```python
from build123d import *

# Parameters (mm, degrees)
CROQUIS1_W              = 160
CROQUIS1_H              = 400
SALIENTE_EXTRUIR1_DEPTH = 400
REDONDEO1_R             = 5
CROQUIS2_R              = 15
CROQUIS2_R_2            = 5
CROQUIS2_W              = 150
CROQUIS2_H              = 40
CROQUIS2_W_2            = 105.514825976
CROQUIS2_H_2            = 8
CORTAR_EXTRUIR1_DEPTH   = 2
CROQUIS3_R              = 12.203694642
CROQUIS3_R_2            = 4.521298069
SALIENTE_EXTRUIR2_DEPTH = 5
CROQUIS4_W              = 380
CROQUIS4_H              = 380
CORTAR_EXTRUIR2_DEPTH   = 2
CROQUIS5_W              = 380
CROQUIS5_H              = 380
CORTAR_EXTRUIR3_DEPTH   = 2


with BuildPart() as part:
    # Croquis1 → Saliente-Extruir1 (new body)
    with BuildSketch(Plane.XY):
        Rectangle(CROQUIS1_W, CROQUIS1_H)
    extrude(amount=-SALIENTE_EXTRUIR1_DEPTH)

    # Redondeo1
    redondeo1_edges = [part.edges().sort_by_distance(p)[0] for p in [
        (80, 0, -400),
        (0, 200, -400),
        (-80, 0, -400),
        (0, 200, 0),
        (80, 0, 0),
        (0, -200, 0),
        (-80, 0, 0),
        (0, -200, -400),
        (-80, 200, -200),
        (80, 200, -200),
        (80, -200, -200),
        (-80, -200, -200),
    ]]
    fillet(redondeo1_edges, radius=REDONDEO1_R)

    # Croquis2 → Cortar-Extruir1 (cut)
    with BuildSketch(Plane.XY):
        with Locations((-42.906419047, -77.137880051)):
            Circle(CROQUIS2_R)
        with Locations((-10.118013228, -77.137880051)):
            Circle(CROQUIS2_R_2)
        with Locations((0, 175)):
            Rectangle(CROQUIS2_W, CROQUIS2_H)
        with Locations((0, 125)):
            Rectangle(CROQUIS2_W, CROQUIS2_H)
        with Locations((0, 35)):
            Rectangle(CROQUIS2_W, CROQUIS2_H)
        with Locations((-0.46526055, -176)):
            Rectangle(CROQUIS2_W_2, CROQUIS2_H_2)
        with Locations((-0.46526055, -158)):
            Rectangle(CROQUIS2_W_2, CROQUIS2_H_2)
        with Locations((-0.46526055, -140)):
            Rectangle(CROQUIS2_W_2, CROQUIS2_H_2)
    extrude(amount=-CORTAR_EXTRUIR1_DEPTH, mode=Mode.SUBTRACT)

    # Croquis3 → Saliente-Extruir2 (add)
    with BuildSketch(Plane.XY.offset(-2)):
        with Locations((-42.906419047, -77.137880051)):
            Circle(CROQUIS3_R)
        with Locations((-10.118013228, -77.137880051)):
            Circle(CROQUIS3_R_2)
    extrude(amount=SALIENTE_EXTRUIR2_DEPTH)

    # Croquis4 → Cortar-Extruir2 (cut)
    with BuildSketch(Plane.ZY.offset(80)):
        with Locations((-200, 0)):
            Rectangle(CROQUIS4_W, CROQUIS4_H)
    extrude(amount=-CORTAR_EXTRUIR2_DEPTH, mode=Mode.SUBTRACT)

    # Croquis5 → Cortar-Extruir3 (cut)
    with BuildSketch(Plane(origin=(80, 0, 0), x_dir=(0, 0, -1), z_dir=(1, 0, 0))):
        with Locations((200, 0)):
            Rectangle(CROQUIS5_W, CROQUIS5_H)
    extrude(amount=-CORTAR_EXTRUIR3_DEPTH, mode=Mode.SUBTRACT)


solid = part.part
```
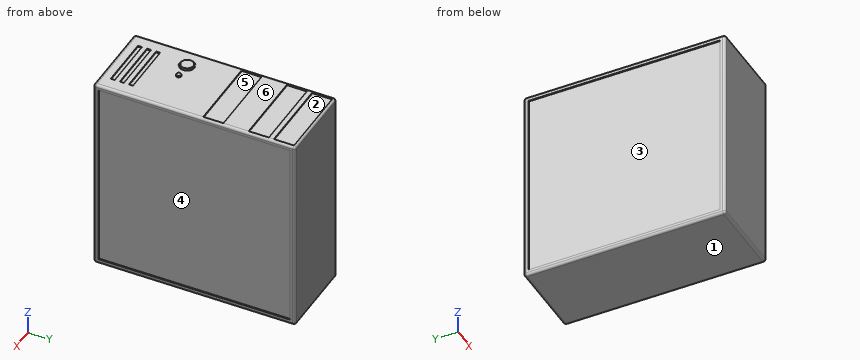
The model under review builds one solid part; all positions refer to its coordinate system, in mm. Face numbers are marked on the shaded views. A direction names the side the tool comes from. Give positions to 0.01 mm unless a question says otherwise; leave off trailing zeros. Write each loop counter-clockwise with the first axis right and the second up, starting at its lowest first coordinate (ties: lowest second). Pieces come first, ordered by that corner, then holes. Notation, with made-up numbers: (-25.5, 46.25) - (1.5, 46.25) arc R18 ccw to (1.5, 57.25) - close; hole circle Ø7 at (84, 38.25). An arc over 180 degrees is marked (long way). Answer in a Markdown table with one row per item. Add a question column.
1. We need section A-A on z = -314. Write out the cut boundary in (x, y).
2. Wall thickness on line 1 along X through (y, z) = (-155, -345); line 2 along Z through (x, y) = (23, -45); line 3 along Z through (x, y) = (9, 138.5): over which ranges is each line inside the solid? List them lowest first. Write a range as [from, to].
3. We need section B-B on y = 94.5. Write out the cut boundary in (x, z).
4. Tool access review of the marked faces 4, 5 and 6: name each direction out of +Z, -Z, +X, -X, +Y, -Y from which nothing blocks a thin tool from reaching the whole face with its end or side.
5. We need section C-C on y = 25.5. Write out the cut boundary in (x, z), then the cut area to 3 significant figures.
6. Insertion check: P1, Ø1, axis at y = -27.5, z = -190, coming from the -X side; P2, Ø1, axis at x = 79, y = 70, coming from the +Z side; P3, Ø2, axis at y = 176, z = -1.5, coming from the -X side. Each pin has a flat end and moves straight along its axis. Give the tip position at first contact, or say it passes through.
7. Draft analysis for pull direction X (two halves, no side actions). For the marked faces 1, 2 and 3, state which applies: +X half, -X half, draft (parallel to the pull), parting line (faces both ways), or undercut.
Ans:
| question | item | result |
|---|---|---|
| 1 | outline | (-80, -195) arc R5 ccw to (-75, -200) - (75, -200) arc R5 ccw to (80, -195) - (80, -190) - (78, -190) - (78, 190) - (80, 190) - (80, 195) arc R5 ccw to (75, 200) - (-75, 200) arc R5 ccw to (-80, 195) - (-80, 190) - (-78, 190) - (-78, -190) - (-80, -190) - close |
| 2 | line 1 | x = [-78, 78] |
| 2 | line 2 | z = [-400, 0] |
| 2 | line 3 | z = [-400, -2] |
| 3 | outline | (-80, -395) arc R5 ccw to (-75, -400) - (75, -400) arc R5 ccw to (80, -395) - (80, -390) - (78, -390) - (78, -10) - (80, -10) - (80, -5) arc R5 ccw to (75, 0) - (-75, 0) arc R5 ccw to (-80, -5) - (-80, -10) - (-78, -10) - (-78, -390) - (-80, -390) - close |
| 4 | face 4 | +X |
| 4 | face 5 | +Z |
| 4 | face 6 | +Z, +X, -X, +Y |
| 5 | outline | (-80, -395) arc R5 ccw to (-75, -400) - (75, -400) arc R5 ccw to (80, -395) - (80, -390) - (78, -390) - (78, -10) - (80, -10) - (80, -5) arc R5 ccw to (75, 0) - (75, -2) - (-75, -2) - (-75, 0) arc R5 ccw to (-80, -5) - (-80, -10) - (-78, -10) - (-78, -390) - (-80, -390) - close |
| 5 | area | 62,200 mm^2 |
| 6 | P1 | stops at x = -78 |
| 6 | P2 | stops at z = -1.43 |
| 6 | P3 | stops at x = -79.33 |
| 7 | face 1 | draft |
| 7 | face 2 | undercut |
| 7 | face 3 | -X half |
